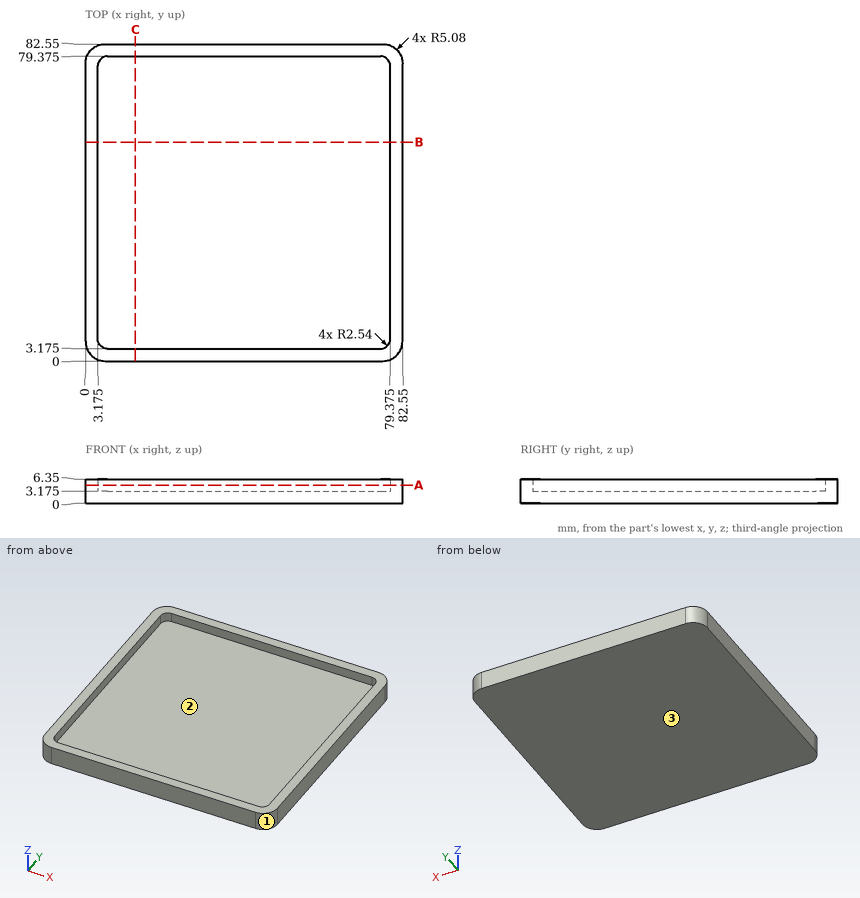
Input: dimensioned drawing with shaded views. Units: mm. Origin: part minimum x, y, z. Round coordinates to 2 decimals unless told otherwise and drop trailing zeros. Order: outer loops, then holes, each group sorted by start corner. A loop starts at its lowest first (then second) coordinate and runs counter-clockwise, first axis right, second up. Notation, with made-up numbers: M 41,17.5 L 72,17.5 A18 ccw 72,49.5 Z; hole C 55.25,-31.75 d5. An arc over 180 degrees is marked long. Use one line per item in the form item = value. Start each with the question number.
Q1. Material intervals for line 1 (X direction, y = 70, z = 5.5) (3 decimals); line 2 (Z direction, x = 32.5, y = 31) (3 decimals), sorted ascending. Write a range as [from, to].
Q2. Mould query, pull axis X, two halves, no side actions, for the marked faces 1, 2 and 3. Classes: +X half, -X half, draft (parallel to the pull), parting line (faces both ways), or undercut.
Q3. Cut plane A-A (z = 4.75). Return loops of the section in (x, y) (3 decimals).
Q4. Cut plane B-B (y = 57). Return loops of the section in (x, z) (3 decimals).
Q5. Pin query (flat end, axial travel): pin 1 Ø4 at (x, y) = (57, 23) entering from +Z (3 decimals). Return the tip coordinate at first contact, or that it passes through.
Geometry results:
q1.line_1 = [0, 3.175], [79.375, 82.55]
q1.line_2 = [0, 3.175]
q2.face_1 = +X half
q2.face_2 = undercut
q2.face_3 = draft
q3.outline = M 0,5.08 A5.08 ccw 5.08,0 L 77.47,0 A5.08 ccw 82.55,5.08 L 82.55,77.47 A5.08 ccw 77.47,82.55 L 5.08,82.55 A5.08 ccw 0,77.47 Z; hole M 3.175,5.715 A2.54 ccw 5.715,3.175 L 76.835,3.175 A2.54 ccw 79.375,5.715 L 79.375,76.835 A2.54 ccw 76.835,79.375 L 5.715,79.375 A2.54 ccw 3.175,76.835 Z
q4.outline = M 0,0 L 82.55,0 L 82.55,6.35 L 79.375,6.35 L 79.375,3.175 L 3.175,3.175 L 3.175,6.35 L 0,6.35 Z
q5.pin_1 = 3.175
